Design review of the part shown in the three views and the two pictorial views. Dimensions are in mm from the part's minimum x, y and z. A direction names the side the tool comes from. Give positions to 0.01 mm unless a question says otherwise; leave off trailing zeros. Loops run counter-clockwise (first coordinate to the right, second up) from the corner with the lowest first, then second, coordinate; pieces in that order, holes last. Notation, with made-up numbers: (72, 58.25) - (104, 58.25) arc R6 cw to (104, 68.25) - close; hole circle Ø10 at (51.5, -23.75). An arc over 180 degrees is marked (long way). Answer as a JSON object with one key per item and string values.
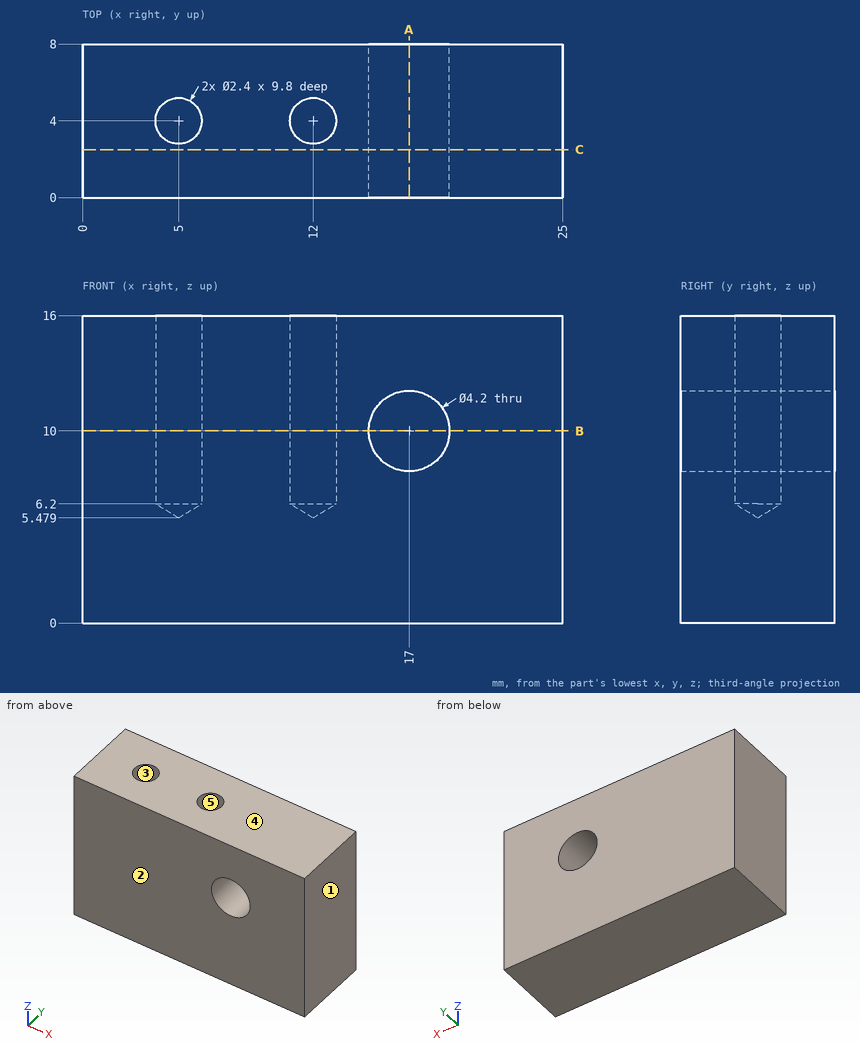
Q1. To check wall thickness, follow probe 1 along X at (y, z) = (4, 13); probe 2 along Y at (x, z) = (12, 12.75); probe 3 along Z at (x, y) = (17, 6.5). State the ranges of each line that lie inside material, in increasing order. Write a range as [from, to].
Results:
{"probe 1": "x = [0, 3.8], [6.2, 10.8], [13.2, 25]", "probe 2": "y = [0, 2.8], [5.2, 8]", "probe 3": "z = [0, 7.9], [12.1, 16]"}
Q2. Consider section C-C, the plane y = 2.5. State the section outline as (x, z) points, plus the area to 3 significant figures.
Results:
{"outline": "(0, 0) - (25, 0) - (25, 16) - (0, 16) - close; hole circle Ø4.2 at (17, 10)", "area": "386 mm^2"}
Q3. Clearance check with a flat-ended pin moving along its axis: pin 1 Ø1.9 at (x, y) = (12, 4) entering from +Z. State where the tip first meets the part, or that it passes through.
Results:
{"pin 1": "stops at z = 6.05"}
Q4. Consider section A-A, the plane x = 17. State the section outline as (y, z) points.
Results:
{"outline": "(0, 0) - (8, 0) - (8, 7.9) - (0, 7.9) - close; (0, 12.1) - (8, 12.1) - (8, 16) - (0, 16) - close"}
Q5. Consider section B-B, the plane z = 10. State the section outline as (x, y) points.
Results:
{"outline": "(0, 0) - (14.9, 0) - (14.9, 8) - (0, 8) - close; (19.1, 0) - (25, 0) - (25, 8) - (19.1, 8) - close; hole circle Ø2.4 at (5, 4); hole circle Ø2.4 at (12, 4)"}
Q6. The part is to be moulded in two halves that separate along Y. For the marked faces 1, 2 and 3, say which applies: +Y half, -Y half, draft (parallel to the pull), parting line (faces both ways), or undercut.
Results:
{"face 1": "draft", "face 2": "-Y half", "face 3": "undercut"}
Q7. For the marked faces 4 and 5, list the 3-axis set-ups (+Z, -Z, +X, -X, +Y, -Y) from which the entire face can be reached by the end or side of a thin tool; tool diameter is ignored.
Results:
{"face 4": "+Z, +X, -X, +Y, -Y", "face 5": "+Z"}
